Geometry: final body of the model. Coordinates: model frame, mm. A direction names the side the tool comes from. Give positions to 0.01 mm unless a question says otherwise; leave off trailing zeros. Loops run counter-clockwise (first coordinate to the right, second up) from the corner with the lowest first, then second, coordinate; pieces in that order, holes last.
1. Material intervals for line 1 along Y through (x, z) = (1.7, 0.2); line 2 along Y through (x, z) = (0, 0.5); line 3 along Z through (x, y) = (0.05, -11.5), sorted ascending.
2. Draft query along X for faces 3 (the face through (0, -16, 0)), 4 (the face through (0, 0.75, 0)), 5 (the face through (0.07, -8.11, -1.5)). Return one class per face: +X half, -X half, draft (parallel to the pull), parting line (faces both ways), or undercut.
3. First-contact query: P1, Ø1, axis at x = 0, z = -0.5, coming from the +Y side. Flat tip, straight axial feed; report the tip coordinate or a pass-through.
4. Access query for faces 1 (the face through (-1, 1.5, 1)), 2 (the face through (-2, 0, 0)). Directions: +Z, -Z, +X, -X, +Y, -Y. A direction counts if a zero-diameter tool reaches every point of the face in a straight line with its end or side. Return the directions, or none.
5. Section A-A, the plane y = -2.5. Output: boundary loops of the cut face in (x, z).
from build123d import *

# Parameters (mm, degrees)
CUT_EXTRUDE1_DEPTH = 0.75
FILLET1_R          = 0.125


with BuildPart() as part:
    # Sketch1 → Revolve1 (revolve)
    with BuildSketch(Plane(origin=(0, 0, 0), x_dir=(0, 0, -1), z_dir=(1, 0, 0))):
        with BuildLine():
            Line((0, 1.5), (-1.75, 1.5))
            ThreePointArc((-1.75, 1.5), (-2.334912942, 0.942930354), (-2.75, 0.25))
            Line((-2.75, 0.25), (-2.605662433, 0))
            Line((-2.605662433, 0), (-1.5, 0))
            Line((-1.5, 0), (-1.5, -16))
            Line((-1.5, -16), (0, -16))
            Line((0, -16), (0, 1.5))
        make_face()
    revolve(axis=Axis((0, -16, 0), (0, 1, 0)))

    # Sketch2 → Cut-Extrude1 (cut)
    with BuildSketch(Plane(origin=(0, 1.5, 0), x_dir=(1, 0, 0), z_dir=(0, 1, 0))):
        Polygon((0, 1.154700538), (-1, 0.577350269), (-1, -0.577350269), (0, -1.154700538), (1, -0.577350269), (1, 0.577350269), align=None)
    extrude(amount=-CUT_EXTRUDE1_DEPTH, mode=Mode.SUBTRACT)

    # Fillet1
    fillet1_edges = [part.edges().sort_by_distance(p)[0] for p in [
        (0.5, 1.5, -0.866025404),
        (-0.5, 1.5, -0.866025404),
        (-1, 1.5, 0),
        (-0.5, 1.5, 0.866025404),
        (0.5, 1.5, 0.866025404),
        (1, 1.5, 0),
        (0, 1.5, -1.75),
    ]]
    fillet(fillet1_edges, radius=FILLET1_R)


solid = part.part
Answers below:
1. line 1: y = 0 to 1.5
1. line 2: y = -16 to 0.75
1. line 3: z = -1.5 to 1.5
2. face 3: draft
2. face 4: undercut
2. face 5: parting line
3. P1: stops at y = 0.75
4. face 1: +Z, -Z, +X, -X, +Y
4. face 2: -Y
5. outline: circle Ø3 at (0, 0)
